Source: CAD feature listing. Evaluate the final solid. Frame: model axes, mm. Give positions to 0.01 mm unless a question says otherwise; leave off trailing zeros. Order: outer loops, then holes, each group sorted by start corner. A loop starts at its lowest first (then second) coordinate and runs counter-clockwise, first axis right, second up. Notation, with made-up numbers: M -28,77 L 26,77 A32 ccw 26,115 Z; hole C -37.5,7 d9. An arc over 180 degrees is marked long. Use CSV: the item, a comma, the result in double quotes. Start each with the question number.
1. Line query: line 1 along X through (y, z) = (-32, 31); line 2 along X through (y, z) = (30.5, 15); line 3 along Z through (x, y) = (-0.5, -37.5). Output: solid intervals per line, ascending. Write a range as [from, to].
2. Mould query, pull axis X, two halves, no side actions, for faces 1 (the flat face through (41, -46.509, -4)), 2 (the cylindrical face through (7.109, -1.829, -54.145)), 3 (the conical face through (-30.94, -15.57, -9.74)). Classes: released by +X, released by -X, zero draft, split by the parting line, or undercut.
3. Pin query (flat end, axial travel): P1, Ø6, axis at y = -28.5, z = -28.5, coming from the -X side; P2, Ø2, axis at x = -42.5, z = 34.5, coming from the -Y side; P3, Ø4, axis at y = 11, z = -8.5, coming from the -X side; P4, Ø8, axis at x = -28.5, y = -25, coming from the +Z side. Return the tip coordinate at first contact, or that it passes through.
4. Section query B-B, the plane z = 0. Return the cut outline in (x, y), plus the area to 3 significant figures.
5. Section query D-D, the plane y = 10. Return the cut outline in (x, z), plus the area to 3 significant figures.
6. Section query A-A, the plane x = 0. Return the cut outline in (y, z), plus the area to 3 significant figures.
7. Section query C-C, the plane y = -31. Return the cut outline in (x, z).
Autodesk Inventor part; units mm, degrees
ref_plane "YZ Plane" through (0, 0, 0) normal (1, 0, 0) x (0, 1, 0)
ref_plane "XZ Plane" through (0, 0, 0) normal (0, 1, 0) x (-1, 0, 0)
ref_plane "XY Plane" through (0, 0, 0) normal (0, 0, 1) x (1, 0, 0)
sketch "Sketch1" plane through (0, 0, 0) normal (0, 0, 1) x (1, 0, 0)
  line L0 (-68.3895, -51.5874) -> (-9.652, -51.5874) construction
  line L1 (-54.61, 44.1185) -> (-48.3044, 44.1185)
  line L2 (-54.61, 44.1185) -> (-9.6509, 44.1185) construction
  line L3 (-54.61, 44.1185) -> (36.0172, 44.1185) construction
  line L4 (-75.5396, 46.8376) -> (-27.9582, 46.8376) construction
  line L5 (-75.5396, 46.8376) -> (-24.3567, 46.8376) construction
  line L6 (-75.5396, 46.8376) -> (-39.9094, 46.8376) construction
  line L7 (-85.2325, 14.4461) -> (-72.647, 14.4461)
  line L8 (-85.2325, 14.4461) -> (-78.8825, 14.4461)
  line L9 (-47.0755, -46.5087) -> (-40.7255, -46.5087)
  line L10 (-54.61, -46.5087) -> (-47.0755, -46.5087)
  arc A0 (-29.1336, -3.2472) -> (-28.7009, 0.0398) centre (-41.4009, 0.0398) ccw
  line L11 (-72.647, 14.4461) -> (-72.647, -49.0501)
  line L12 (-85.2325, 7.0204) -> (-85.2325, -49.0501)
  line L13 (-78.8825, 7.0204) -> (-85.2325, 7.0204)
  line L14 (-78.8825, 14.4461) -> (-78.8825, 7.0204)
  line L15 (-54.61, 44.1185) -> (-54.61, -46.5087)
  line L16 (-29.1336, -3.2472) -> (-78.2122, -186.4111)
  line L17 (-78.997, -110.2264) -> (-72.647, -110.2264)
  line L18 (-72.647, -141.9758) -> (-66.3058, -141.9758)
  line L19 (-78.997, -110.2264) -> (-78.997, -186.4111)
  line L20 (-72.647, -49.0501) -> (-85.2325, -49.0501)
  line L21 (-72.6469, -48.8475) -> (-59.9469, -48.8475) construction
  line L22 (-85.2325, 26.3534) -> (-71.1236, 26.3534)
  line L23 (-71.1236, 26.3534) -> (-64.7736, 26.3534)
  line L24 (-64.7736, 26.3534) -> (-64.7736, -49.0592)
  line L25 (-64.7736, -49.0592) -> (-64.7736, -112.5592)
  line L26 (-64.7736, -112.5592) -> (-58.4236, -112.5592)
  line L27 (-85.2325, 26.3534) -> (-85.2325, 42.2284)
  line L28 (-85.2325, 42.2284) -> (-78.2952, 42.2284)
  line L29 (-78.2952, 42.2284) -> (-78.2952, 58.1034)
  line L30 (-78.2952, 58.1034) -> (-48.3044, 44.1185)
  line L31 (-77.6767, 58.2932) -> (49.3233, 58.2932) construction
  arc A1 (-28.7009, 0.0398) -> (-48.3044, 44.1185) centre (-75.5766, 5.5909) ccw
  line L32 (-78.997, -186.4111) -> (-78.2122, -186.4111)
  line L33 (-72.6558, -49.0501) -> (-72.647, -49.0501)
  line L34 (-85.2325, 26.3534) -> (-85.2325, 14.4461)
  line L35 (-72.647, -49.0501) -> (-72.647, -110.2264)
  line L36 (-72.647, -110.2264) -> (-72.647, -141.9758)
  line L37 (0, -235.352) -> (0, 107.2341)
  point P0 (0, 0)
  point P1 (-9.6509, 0.0398)
  dimension "d5" = 12.7
  dimension "d7" = 6.35
  dimension "d8" = 105
  dimension "d23" = 76.1847
  dimension "d26" = 31.7495
  dimension "d30" = 90
  dimension "d33" = 6.35
  dimension "d51" = 6.35
  dimension "d54" = 6.35
  dimension "d55" = 15.875
  dimension "d56" = 6.9374
  dimension "d57" = 15.875
  dimension "d60" = 25
  dimension "d62" = 28.7008
  dimension "d63" = 54.61
  dimension "d64" = 6.3056
revolve "Revolution1" add sketch "Sketch1" angle 360 about axis through (0, -10, 0) along (0, 1, 0) contours L1 A1 A0 L16 L9 L10 L15
properties part number "nozzle 8in version 1"
Result set:
1,line 1,"[-44.96, -19.9], [19.9, 44.96]"
1,line 2,"[-52.51, -32.15], [32.15, 52.51]"
1,line 3,"[-54.61, -38.31], [38.31, 54.61]"
2,face 1,"zero draft"
2,face 2,"split by the parting line"
2,face 3,"undercut"
3,P1,"x = -48.29"
3,P2,"y = -46.51"
3,P3,"x = -54.22"
3,P4,"z = 48.81"
4,outline,"M -54.61,-46.51 L -40.73,-46.51 L -29.13,-3.25 A12.7 ccw -28.7,0.04 A47.2 ccw -48.3,44.12 L -54.61,44.12 Z; M 28.7,0.04 A12.7 ccw 29.13,-3.25 L 40.73,-46.51 L 54.61,-46.51 L 54.61,44.12 L 48.3,44.12 A47.2 ccw Z"
4,area,"3,720 mm2"
5,outline,"C 0,0 d109.22; hole C 0,0 d57.16"
5,area,"6,800 mm2"
6,outline,"M -46.51,-54.61 L 44.12,-54.61 L 44.12,-48.3 A47.2 ccw 0.04,-28.7 A12.7 ccw -3.25,-29.13 L -46.51,-40.73 Z; M -46.51,40.73 L -3.25,29.13 A12.7 ccw 0.04,28.7 A47.2 ccw 44.12,48.3 L 44.12,54.61 L -46.51,54.61 Z"
6,area,"3,720 mm2"
7,outline,"C 0,0 d109.22; hole C 0,0 d73.14"
